Geometry: see drawing. Coordinates: mm, zero at the bounding-box minimum. A direction names the side the tool comes from. Coordinates: 2 decimals unless noted, no trailing zeros. Order: outer loops, then holes, each group sorted by start corner. A loop starts at its lowest first (then second) coordinate and runs counter-clockwise, first axis right, second up. Notation, with made-up numbers: (-39, 21.5) -> (-18, 21.5) arc R19 ccw to (-18, 51.5) -> close; hole circle Ø1 at (-13, 10.5). An arc over 180 degrees is marked (long way). Write each question's results on one line, items separated by ' | '.
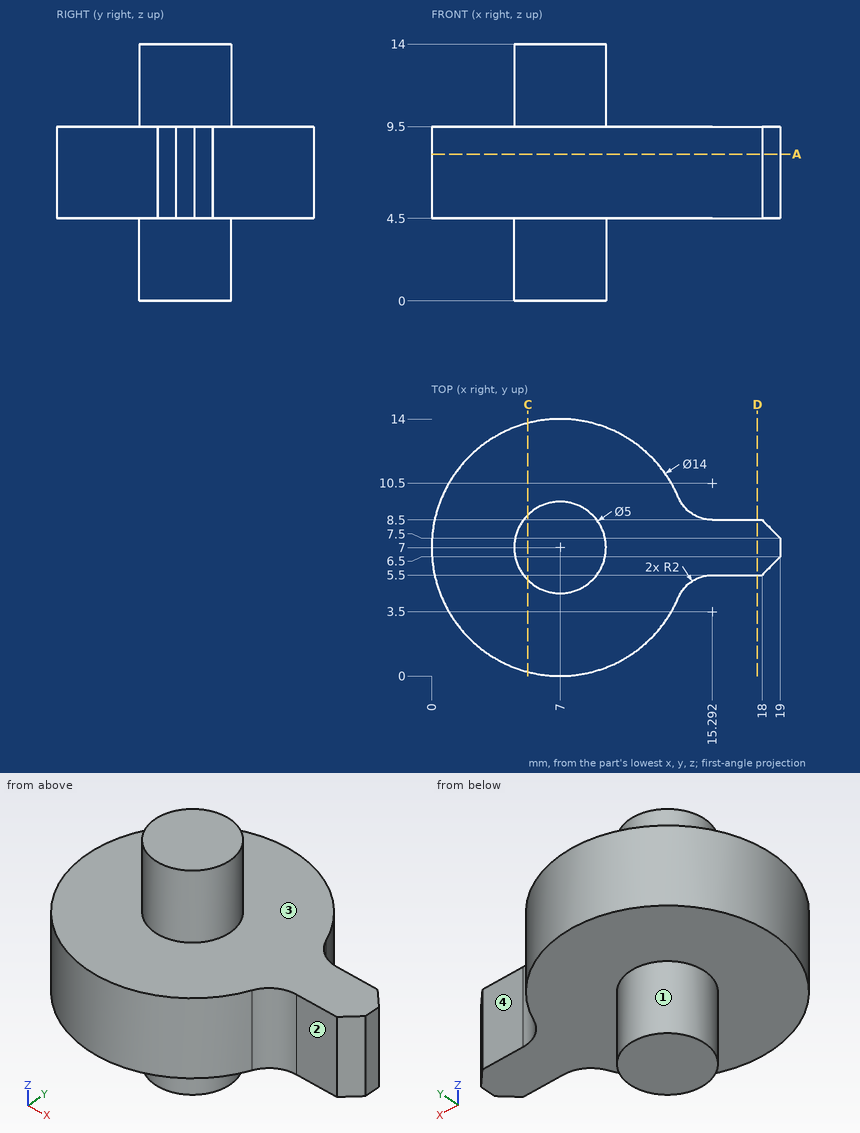
(1) Line query: line 1 along Z through (x, y) = (6.25, 10); line 2 along X through (y, z) = (12, 8.5). Output: solid intervals per line, ascending. Write a range as from..to.
Return value:
line 1: 4.5..9.5 | line 2: 2.1..11.9
(2) Cut plane C-C, the plane x = 5.25. Return loops of the section in (y, z) (1 decimal).
Return value:
outline: (0.2, 4.5) -> (5.2, 4.5) -> (5.2, 0) -> (8.8, 0) -> (8.8, 4.5) -> (13.8, 4.5) -> (13.8, 9.5) -> (8.8, 9.5) -> (8.8, 14) -> (5.2, 14) -> (5.2, 9.5) -> (0.2, 9.5) -> close
(3) Cut plane A-A, the plane z = 8. Return loops of the section in (x, y), plus the area to 3 significant figures.
Return value:
outline: (13.45, 4.28) arc R2 cw to (15.29, 5.5) -> (18, 5.5) -> (19, 6.5) -> (19, 7.5) -> (18, 8.5) -> (15.29, 8.5) arc R2 cw to (13.45, 9.72) arc R7 ccw (long way) to start | area: 169 mm2
(4) Cut plane D-D, the plane x = 17.75. Return loops of the section in (y, z), plus the area to 3 significant figures.
Return value:
outline: (5.5, 4.5) -> (8.5, 4.5) -> (8.5, 9.5) -> (5.5, 9.5) -> close | area: 15.0 mm2
(5) Pin query (flat end, axial travel): P1, Ø1, axis at x = 12, y = 10.5, coming from the -Z side; P2, Ø5, axis at x = 4.5, y = 2, coming from the +Z side; P3, Ø4, axis at x = 10, z = 9, coming from the +Y side. Return the tip coordinate at first contact, or that it passes through.
Return value:
P1: z = 4.5 | P2: z = 9.5 | P3: y = 13.93
(6) Reachability of the marked faces 1, 2, 3 and 4 from +Z, -Z, +X, -X, +Y, -Y: full face, straight path, thin tool, end or side. Return the list, or none.
Return value:
face 1: -Z | face 2: +Z, -Z, +X, -Y | face 3: +Z | face 4: +Z, -Z, +X, +Y
